Can you work these out from the model? Positions are in its coordinate system, mm. Give positions to 0.01 mm unless a question says otherwise; leave off trailing zeros. Loops run counter-clockwise (first coordinate to the right, second up) from the corner with the lowest first, then second, coordinate; pieces in that order, holes last. Notation, with made-up numbers: M 73.25,71.25 L 90.25,71.25 A23 cw 90.25,92.25 Z; hole C -27.5,1.5 d3. An arc over 180 degrees is marked long. Use CSV: the item, a comma, the result in double quotes.
from build123d import *

# Parameters (mm, degrees)
SKETCH1_R               = 2
BOSS_EXTRUDE1_DEPTH     = 20
SKETCH2_R               = 1
CUT_EXTRUDE1_DEPTH      = 3
CUT_EXTRUDE1_DEPTH_BACK = 3
CHAMFER1_SIZE           = 0.5


with BuildPart() as part:
    # Sketch1 → Boss-Extrude1 (new body)
    with BuildSketch(Plane(origin=(0, 0, 0), x_dir=(0, 0, -1), z_dir=(1, 0, 0))):
        Circle(SKETCH1_R)
    extrude(amount=-BOSS_EXTRUDE1_DEPTH)

    # Sketch2 → Cut-Extrude1 (cut, two sides)
    with BuildSketch(Plane.XY) as cut_extrude1_sk:
        with Locations((-16, 0)):
            Circle(SKETCH2_R)
    extrude(amount=CUT_EXTRUDE1_DEPTH, mode=Mode.SUBTRACT)
    extrude(cut_extrude1_sk.sketch, amount=-CUT_EXTRUDE1_DEPTH_BACK, mode=Mode.SUBTRACT)

    # Chamfer1
    chamfer1_edges = [part.edges().sort_by_distance(p)[0] for p in [
        (-20, 0, 2),
    ]]
    chamfer(chamfer1_edges, length=CHAMFER1_SIZE)

    # Sketch3 → Revolve1 (revolve)
    with BuildSketch(Plane(origin=(0, 0, 0), x_dir=(1, 0, 0), z_dir=(0, 1, 0))):
        with BuildLine():
            Line((2.757385023, 0), (0, 0))
            Line((0, 0), (0, 3.5))
            ThreePointArc((0, 3.5), (1.985229955, 2.227844932), (2.757385023, 0))
        make_face()
    revolve(axis=Axis((3.35333719, 0, 0), (-1, 0, 0)))


solid = part.part
Q1. I want a section at B-B, the plane z = 0. Please give me the cut outline in (x, y), then the cut area to 3 significant figures.
Model answer:
outline,"M -20,-1.5 L -19.5,-2 L 0,-2 L 0,-3.5 A3.6 ccw 0,3.5 L 0,2 L -19.5,2 L -20,1.5 Z; hole C -16,0 d2"
area,"91.0 mm2"
Q2. I want a section at A-A, the plane y = 0. Please give me the cut outline in (x, z), then the cut area to 3 significant figures.
Model answer:
outline,"M -20,-1.5 L -19.5,-2 L -17,-2 L -17,2 L -19.5,2 L -20,1.5 Z; M -15,-2 L 0,-2 L 0,-3.5 A3.6 ccw 0,3.5 L 0,2 L -15,2 Z"
area,"86.1 mm2"
Q3. I want a section at C-C, the plane x = -16. Please give me the cut outline in (y, z), then the cut area to 3 significant figures.
Model answer:
outline,"M -1,-1.73 L -1,1.73 A2 ccw Z; M 1,-1.73 A2 ccw 1,1.73 Z"
area,"4.91 mm2"
Q4. I want a section at D-D, the plane x = -11.75. Please give me the cut outline in (y, z).
Model answer:
outline,"C 0,0 d4"
Q5. If we mould it in two halves opening along X, with no side actions, what happens to faces 1 (the cylindrical face through (-15.46, 0.84, 0.03)), 2 (the flat face through (0, 2, 2)), 3 (the cylindrical face through (-10, 0, 2))? For each: released by +X, released by -X, zero draft, split by the parting line, or undercut.
Model answer:
face 1,"undercut"
face 2,"released by -X"
face 3,"zero draft"
Q6. I'm going to push flat-ended pins straight in: P1, Ø1.5, axis at x = -12.5, z = -0.5, coming from the +Y side; P2, Ø4, axis at x = -16, y = -0.5, coming from the -Z side; P3, Ø2.5, axis at x = -16, y = 0, coming from the +Z side. Where does each tip first touch, or does it pass through?
Model answer:
P1,"y = 2"
P2,"z = -2"
P3,"z = 2"
Q7. Please list where these lines run through material, in increasing order: L1, parallel to X at y = 0, z = -0.25; L2, parallel to Y at x = -16, z = -1.2; L3, parallel to X at y = 0, z = 1.05. Write a range as from..to.
Model answer:
L1,"-20..-17, -15..2.75"
L2,"-1.6..-1, 1..1.6"
L3,"-20..-17, -15..2.6"
